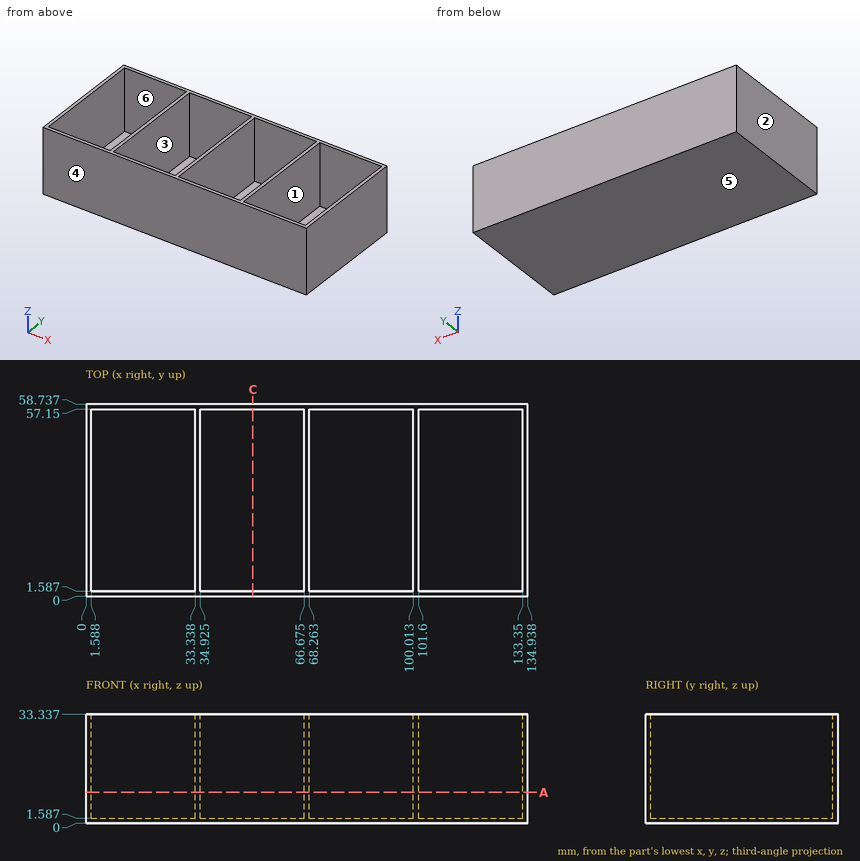
Could you check a few things on this drawing? It's one solid part, dimensions in mm from its lowest x, y, z. A direction names the side the tool comes from. Coordinates: 2 decimals unless noted, no trailing zeros. Write each loop counter-clockwise with the first axis right and the second up, starting at its lowest first coordinate (ties: lowest second). Pieces come first, ordered by that corner, then holes. Notation, with made-up numbers: M -9,69 L 40,69 A22 ccw 40,108 Z; hole C 28.5,-21 d8. An arc over 180 degrees is marked long. Answer as CSV lines item,"result". Start each with the question number.
Q1. Will this pin go through, and if not, where does the flat tip stop? pin 1 Ø8 at (x, y) = (16.5, 28.5) entering from +Z.
Q2. Suppose I cut it at A-A, the plane z = 9.5. State how many separate pieces and enclosed holes the cut face has.
Q3. If we mould it in two halves opening along Y, with no side actions, what happens to the marked faces 3, 4, 5 and 6? For each: pulls with the +Y half, pulls with the -Y half, needs draft (parallel to the pull), parting line crosses it, or undercut.
Q4. I need wall thicknesses on probe 1 along Y at (x, z) = (64.5, 13); probe 2 along Z at (x, y) = (123.5, 17.5). Which ranges of each line are inside material? Lowest first, please. Write a range as [from, to].
Q5. Suppose I cut it at C-C, the plane x = 51. List the corners of the cut face in (y, z) for me, then the cut area to 3 significant figures.
Q6. For the marked faces 1 and 2, which set-ups out of +Z, -Z, +X, -X, +Y, -Y let a thin tool reach every point of the face, with its end or its side?
Entries:
1,pin 1,"stops at z = 1.59"
2,separate pieces,"1"
2,enclosed holes,"4"
3,face 3,"undercut"
3,face 4,"pulls with the -Y half"
3,face 5,"needs draft"
3,face 6,"undercut"
4,probe 1,"y = [0, 1.59], [57.15, 58.74]"
4,probe 2,"z = [0, 1.59]"
5,outline,"M 0,0 L 58.74,0 L 58.74,33.34 L 57.15,33.34 L 57.15,1.59 L 1.59,1.59 L 1.59,33.34 L 0,33.34 Z"
5,area,"194 mm²"
6,face 1,"+Z"
6,face 2,"+Z, -Z, -X, +Y, -Y"
